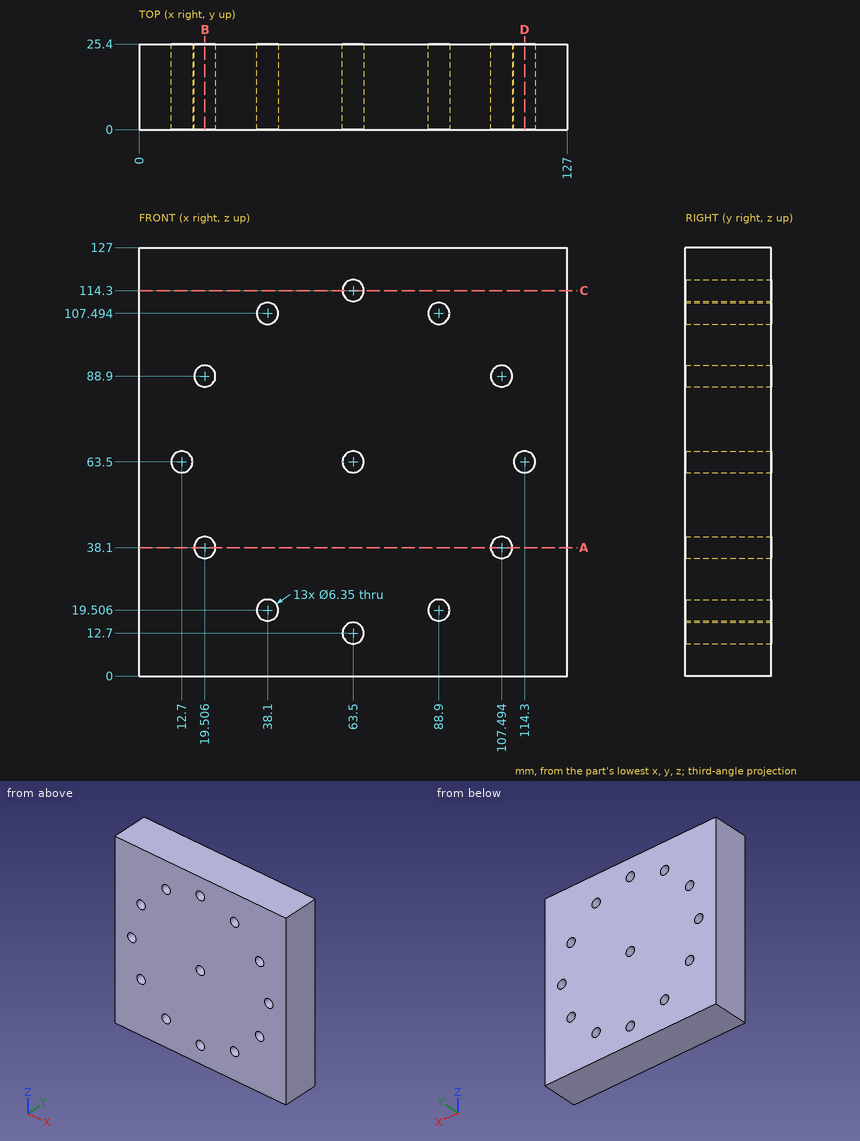
Study the drawing (mm; zero at the part's minimum x, y, z) and answer. Give positions to 0.01 mm unless a question says otherwise; leave off trailing zeros. Order: outer loops, then holes, each group sorted by start corner. A loop starts at its lowest first (then second) coordinate and runs counter-clockwise, first axis right, second up.
1. Straight lines are drawn through the part: L1, parallel to Z at x = 88.9, y = 15.75; L2, parallel to Z at x = 63.5, y = 5.5 (3 decimals); L3, parallel to X at y = 20.75, z = 114. For each, find the intervals that lie inside material, in ascending order.
Result sheet:
L1: z = 0 to 16.33, 22.68 to 104.32, 110.67 to 127
L2: z = 0 to 9.525, 15.875 to 60.325, 66.675 to 111.125, 117.475 to 127
L3: x = 0 to 60.34, 66.66 to 127
2. Section C-C, the plane z = 114.3 is taken. Determine the outline of the cut face in (x, y) (3 decimals).
Result sheet:
outline: (0, 0) - (60.325, 0) - (60.325, 25.4) - (0, 25.4) - close; (66.675, 0) - (127, 0) - (127, 25.4) - (66.675, 25.4) - close
3. Section A-A, the plane z = 38.1 is taken. Determine the outline of the cut face in (x, y).
Result sheet:
outline: (0, 0) - (16.33, 0) - (16.33, 25.4) - (0, 25.4) - close; (22.68, 0) - (104.32, 0) - (104.32, 25.4) - (22.68, 25.4) - close; (110.67, 0) - (127, 0) - (127, 25.4) - (110.67, 25.4) - close
4. Section D-D, the plane x = 114.3 is taken. Determine the outline of the cut face in (y, z) (3 decimals).
Result sheet:
outline: (0, 0) - (25.4, 0) - (25.4, 60.325) - (0, 60.325) - close; (0, 66.675) - (25.4, 66.675) - (25.4, 127) - (0, 127) - close
5. Section B-B, the plane x = 19.5 is taken. Determine the outline of the cut face in (y, z) (3 decimals), and give its area (3 significant figures).
Result sheet:
outline: (0, 0) - (25.4, 0) - (25.4, 34.925) - (0, 34.925) - close; (0, 41.275) - (25.4, 41.275) - (25.4, 85.725) - (0, 85.725) - close; (0, 92.075) - (25.4, 92.075) - (25.4, 127) - (0, 127) - close
area: 2,900 mm2
